```python
from build123d import *

# Parameters (mm, degrees)
SKETCH_1_R          = 25
EXTRUDE_2_DEPTH     = 3
SKETCH_2_R          = 18
CUT_EXTRUDE_1_DEPTH = 36.482389998
CHAMFER_1_SIZE      = 0.5
CHAMFER_1_SIZE2     = 0.288675135


with BuildPart() as part:
    # 草图1 → 拉伸2 (new body)
    with BuildSketch(Plane.XY):
        Circle(SKETCH_1_R)
    extrude(amount=EXTRUDE_2_DEPTH)

    # 草图2 → 切除-拉伸1 (cut, through all)
    with BuildSketch(Plane.XY.offset(3)):
        Circle(SKETCH_2_R)
    extrude(amount=-CUT_EXTRUDE_1_DEPTH, mode=Mode.SUBTRACT)

    # 倒角1
    chamfer_1_edges = [part.edges().sort_by_distance(p)[0] for p in [
        (-25, 0, 3),
    ]]
    chamfer_1_side = [part.faces().sort_by_distance(p)[0] for p in [
        (-25, 0, 1.5),
    ]]
    chamfer(chamfer_1_edges, length=CHAMFER_1_SIZE, length2=CHAMFER_1_SIZE2, reference=chamfer_1_side[0])


solid = part.part
```
Build history of the part. All positions in model axes, mm. Coordinates: 2 decimals unless noted, no trailing zeros. Write each loop counter-clockwise with the first axis right and the second up, starting at its lowest first coordinate (ties: lowest second). Pieces come first, ordered by that corner, then holes.
1. Pull direction X, two halves, no side cores. Call faces 1 (the cylindrical face through (23.846, 7.509, 1.232)), 2 (the flat face through (11, -16, 0)), 3 (the cylindrical face through (-2.343, 17.847, 1.521)): released by +X, released by -X, zero draft, split by the parting line, or undercut.
Answer block:
face 1: split by the parting line
face 2: zero draft
face 3: undercut
2. Drill centre lines: probe 1 along Y at (x, z) = (0, 2.25); probe 2 along X at (y, z) = (-12, 0.55); probe 3 along Y at (x, z) = (-2, 1.7). Where is each one in solid material? Low to high.
Answer block:
probe 1: y = -25 to -18, 18 to 25
probe 2: x = -21.93 to -13.42, 13.42 to 21.93
probe 3: y = -24.92 to -17.89, 17.89 to 24.92
3. Band-saw the part on C-C, the plane z = 1.8. Give the cut face in (x, y), and give its area (3 significant figures).
Answer block:
outline: circle Ø50 at (0, 0); hole circle Ø36 at (0, 0)
area: 946 mm2
4. Drop flat-ended pins along their axis: pin 1 (1.5 mm diameter, centred on y = 14, z = 1.5, fed in from -X); pin 2 (10 mm diameter, centred on x = 5, y = -11, fed in from +Z); pin 3 (1 mm diameter, centred on x = 7, z = 2, fed in from +Y). Give the stop position or say it passes through.
Answer block:
pin 1: stops at x = -21.2
pin 2: passes through
pin 3: stops at y = 24.14
5. Band-saw the part on A-A, the plane x = 0. Give the cut face in (y, z).
Answer block:
outline: (-25, 0) - (-18, 0) - (-18, 3) - (-24.71, 3) - (-25, 2.5) - close; (18, 0) - (25, 0) - (25, 2.5) - (24.71, 3) - (18, 3) - close
